Verification items for the finished model (mm, model axes). Face numbers are marked on the shaded views. A direction names the side the tool comes from. Coordinates: 2 decimals unless noted, no trailing zeros. Order: outer loops, then holes, each group sorted by start corner. A loop starts at its lowest first (then second) coordinate and runs counter-clockwise, first axis right, second up. Notation, with made-up numbers: M -8.75,-28 L 34.25,-28 A19 cw 34.25,-8 Z; hole C 2,87 d1. An arc over 180 degrees is marked long. Write item = value, one per line.
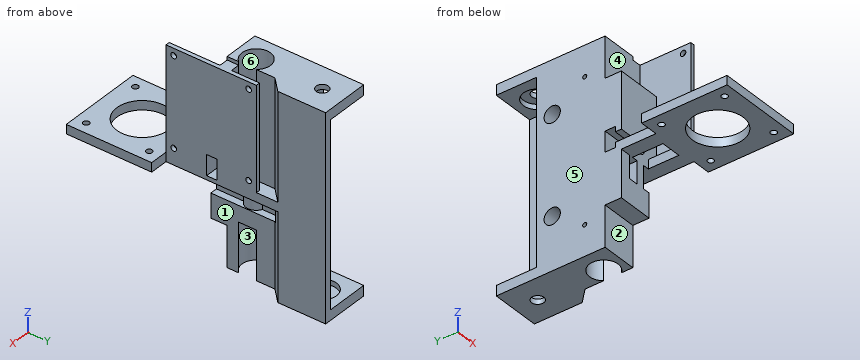
```python
from build123d import *

# Parameters (mm, degrees)
SKETCH1_R               = 7
BOSS_EXTRUDE1_DEPTH     = 50
SKETCH2_R               = 4
CUT_EXTRUDE1_DEPTH      = 17
SKETCH3_W               = 5
SKETCH3_H               = 19.75
BOSS_EXTRUDE2_DEPTH     = 21
SKETCH4_R               = 7
CUT_EXTRUDE4_DEPTH      = 47.5
SKETCH6_R               = 7
SKETCH6_R_2             = 5
BOSS_EXTRUDE3_DEPTH     = 26
CUT_EXTRUDE5_REACH      = 63.576
CUT_EXTRUDE5_END_RADIUS = 7
SKETCH7_R               = 1
CUT_EXTRUDE6_DEPTH      = 102.812634392
CUT_EXTRUDE6_DEPTH_BACK = 102.812634392
SKETCH8_R               = 3
CUT_EXTRUDE7_DEPTH      = 105.209224747
BOSS_EXTRUDE4_DEPTH     = 17.5
CUT_EXTRUDE8_DEPTH      = 78.886134918
SKETCH12_W              = 5
SKETCH12_H              = 11.1
CUT_EXTRUDE9_DEPTH      = 67.234904034
BOSS_EXTRUDE5_REACH     = 82.164
SKETCH13_W              = 6.5
SKETCH13_H              = 4.5
SKETCH14_W              = 2.5
SKETCH14_H              = 5
CUT_EXTRUDE10_DEPTH     = 64.354656605
SKETCH16_R              = 12.5
SKETCH16_R_2            = 1.5
BOSS_EXTRUDE8_DEPTH     = 4.5
SKETCH18_R              = 1.375
BOSS_EXTRUDE9_DEPTH     = 2
BOSS_EXTRUDE10_REACH    = 112.68


with BuildPart() as part:
    # Sketch1 → Boss-Extrude1 (new, symmetric)
    with BuildSketch(Plane.XY):
        Polygon((-12, 7), (9, 7), (9, 26.75), (12, 26.75), (12, -26.75), (-12, -26.75), align=None)
        with Locations((0, -16.75)):
            Circle(SKETCH1_R, mode=Mode.SUBTRACT)
    extrude(amount=BOSS_EXTRUDE1_DEPTH, both=True)

    # Sketch2 → Cut-Extrude1 (cut)
    with BuildSketch(Plane.ZY.offset(12)):
        with Locations((-24.1, -0.75)):
            Circle(SKETCH2_R)
        with Locations((24.1, -0.75)):
            Circle(SKETCH2_R)
    extrude(amount=-CUT_EXTRUDE1_DEPTH, mode=Mode.SUBTRACT)

    # Sketch3 → Boss-Extrude2 (add, through all)
    with BuildSketch(Plane.ZY.offset(-9)):
        with Locations((-47.5, 16.875)):
            Rectangle(SKETCH3_W, SKETCH3_H)
        with Locations((47.5, 16.875)):
            Rectangle(SKETCH3_W, SKETCH3_H)
    extrude(amount=BOSS_EXTRUDE2_DEPTH)

    # Sketch4 → Cut-Extrude4 (cut, symmetric)
    with BuildSketch(Plane.XY):
        with Locations((0, 15.75)):
            Circle(SKETCH4_R)
    extrude(amount=CUT_EXTRUDE4_DEPTH, both=True, mode=Mode.SUBTRACT)

    # Sketch6 → Boss-Extrude3 (add, symmetric)
    with BuildSketch(Plane.XY):
        with Locations((0, -16.75)):
            Circle(SKETCH6_R)
        with Locations(Location((0, -16.75, 0), (0, 0, 180))):
            Circle(SKETCH6_R_2, mode=Mode.SUBTRACT)
    extrude(amount=BOSS_EXTRUDE3_DEPTH, both=True)

    # Cut-Extrude5: up to this cylinder (the profile starts outside it)
    cut_extrude5_end = Plane(origin=(0, -16.75, 0), z_dir=(0, 0, -1)) * Cylinder(CUT_EXTRUDE5_END_RADIUS, 212.152, mode=Mode.PRIVATE)
    # Sketch7 → Cut-Extrude5 (cut, up to the surface)
    with BuildSketch(Plane.ZY.offset(12), mode=Mode.PRIVATE) as cut_extrude5_sk1:
        with Locations((-35, -16.75)):
            Circle(SKETCH7_R)
    cut_extrude5_tool1 = extrude(cut_extrude5_sk1.sketch, amount=-CUT_EXTRUDE5_REACH, mode=Mode.PRIVATE) - cut_extrude5_end
    add(cut_extrude5_tool1.solids().sort_by_distance((-12, -16.75, -35))[0], mode=Mode.SUBTRACT)
    # Sketch7 → Cut-Extrude5 (cut, up to the surface)
    with BuildSketch(Plane.ZY.offset(12), mode=Mode.PRIVATE) as cut_extrude5_sk2:
        with Locations((35, -16.75)):
            Circle(SKETCH7_R)
    cut_extrude5_tool2 = extrude(cut_extrude5_sk2.sketch, amount=-CUT_EXTRUDE5_REACH, mode=Mode.PRIVATE) - cut_extrude5_end
    add(cut_extrude5_tool2.solids().sort_by_distance((-12, -16.75, 35))[0], mode=Mode.SUBTRACT)

    # Sketch8 → Cut-Extrude6 (cut, two sides: drawn at the far end of the back side and taken through both)
    with BuildSketch(Plane(origin=(0, 0, 47.5), x_dir=(-1, 0, 0), z_dir=(0, 0, -1)).offset(-CUT_EXTRUDE6_DEPTH_BACK)):
        with Locations((0, 15.75)):
            Circle(SKETCH8_R)
    extrude(amount=CUT_EXTRUDE6_DEPTH + CUT_EXTRUDE6_DEPTH_BACK, mode=Mode.SUBTRACT)

    # Sketch9 → Cut-Extrude7 (cut, through all)
    with BuildSketch(Plane.XY.offset(50)):
        Polygon((5.5, -3.25), (12, 3.25), (12, -26.75), (5.5, -26.75), align=None)
    extrude(amount=-CUT_EXTRUDE7_DEPTH, mode=Mode.SUBTRACT)

    # Sketch10 → Boss-Extrude4 (add)
    with BuildSketch(Plane.ZY.offset(12)):
        Polygon((-5, -26.75), (-5, -31.75), (5, -31.75), (5, -26.75), (30, -26.75), (30, -34.75), (-30, -34.75), (-30, -26.75), align=None)
    extrude(amount=-BOSS_EXTRUDE4_DEPTH)

    # Sketch11 → Cut-Extrude8 (cut, through all)
    with BuildSketch(Plane(origin=(0, -31.75, 0), x_dir=(1, 0, 0), z_dir=(0, 1, 0))):
        with BuildLine():
            Line((0, 2.5), (-12, 2.5))
            Line((-12, 2.5), (-12, -2.5))
            Line((-12, -2.5), (0, -2.5))
            ThreePointArc((0, -2.5), (2.5, 0), (0, 2.5))
        make_face()
    extrude(amount=-CUT_EXTRUDE8_DEPTH, mode=Mode.SUBTRACT)

    # Sketch12 → Cut-Extrude9 (cut, through all)
    with BuildSketch(Plane(origin=(0, 7, 0), x_dir=(1, 0, 0), z_dir=(0, 1, 0))):
        with Locations((4.5, 12.55)):
            Rectangle(SKETCH12_W, SKETCH12_H)
        with Locations((-4.5, 12.55)):
            Rectangle(SKETCH12_W, SKETCH12_H)
    extrude(amount=-CUT_EXTRUDE9_DEPTH, mode=Mode.SUBTRACT)

    # Sketch13 → Boss-Extrude5 (add, up to next)
    with BuildSketch(Plane.XZ.offset(34.75), mode=Mode.PRIVATE) as boss_extrude5_sk1:
        with Locations((8.75, -4.75)):
            Rectangle(SKETCH13_W, SKETCH13_H)
    boss_extrude5_tool1 = extrude(boss_extrude5_sk1.sketch, amount=-BOSS_EXTRUDE5_REACH, mode=Mode.PRIVATE) - part.part
    add(boss_extrude5_tool1.solids().sort_by_distance((8.75, -34.75, -4.75))[0])

    # Sketch14 → Cut-Extrude10 (cut, through all)
    with BuildSketch(Plane.ZY.offset(-5.5)):
        with Locations((-3.75, -29.25)):
            Rectangle(SKETCH14_W, SKETCH14_H)
    extrude(amount=-CUT_EXTRUDE10_DEPTH, mode=Mode.SUBTRACT)

    # Sketch16 → Boss-Extrude8 (add)
    with BuildSketch(Plane(origin=(0, 0, -7), x_dir=(-1, 0, 0), z_dir=(0, 0, -1))):
        Polygon((-12, -34.75), (-5, -34.75), (-5, -49.75), (5, -49.75), (5, -34.75), (12, -34.75), (12, -51.75), (21, -51.75), (21, -93.75), (-21, -93.75), (-21, -51.75), (-12, -51.75), align=None)
        with Locations((0, -72.75)):
            Circle(SKETCH16_R, mode=Mode.SUBTRACT)
        with Locations((-15.5, -57.25)):
            Circle(SKETCH16_R_2, mode=Mode.SUBTRACT)
        with Locations((15.5, -57.25)):
            Circle(SKETCH16_R_2, mode=Mode.SUBTRACT)
        with Locations((15.5, -88.25)):
            Circle(SKETCH16_R_2, mode=Mode.SUBTRACT)
        with Locations((-15.5, -88.25)):
            Circle(SKETCH16_R_2, mode=Mode.SUBTRACT)
    extrude(amount=-BOSS_EXTRUDE8_DEPTH)

    # Sketch18 → Boss-Extrude9 (add)
    with BuildSketch(Plane(origin=(12, 0, 0), x_dir=(0, 0, -1), z_dir=(1, 0, 0))):
        Polygon((2.5, -51.75), (-48.3, -51.75), (-48.3, -7.3), (2.5, -7.3), (2.5, -26.75), (-5, -26.75), (-5, -31.75), (2.5, -31.75), align=None)
        with Locations((-44.81, -11.11)):
            Circle(SKETCH18_R, mode=Mode.SUBTRACT)
        with Locations((-0.99, -47.94)):
            Circle(SKETCH18_R, mode=Mode.SUBTRACT)
        with Locations((-44.81, -47.94)):
            Circle(SKETCH18_R, mode=Mode.SUBTRACT)
        with Locations((-1.63, -11.11)):
            Circle(SKETCH18_R, mode=Mode.SUBTRACT)
    extrude(amount=-BOSS_EXTRUDE9_DEPTH)

    # Sketch20 → Boss-Extrude10 (add, up to next)
    with BuildSketch(Plane.ZY.offset(-10), mode=Mode.PRIVATE) as boss_extrude10_sk1:
        Polygon((-2.5, -31.75), (-2.5, -34.75), (30, -34.75), (30, -26.75), (48.3, -26.75), (48.3, -21.080127019), (-2.5, -21.080127019), (-2.5, -26.75), (5, -26.75), (5, -31.75), align=None)
    boss_extrude10_tool1 = extrude(boss_extrude10_sk1.sketch, amount=BOSS_EXTRUDE10_REACH, mode=Mode.PRIVATE) - part.part
    add(boss_extrude10_tool1.solids().sort_by_distance((10, -27.004059, 19.830393))[0])


solid = part.part
```
Item 1: Release check for a two-part mould opening along Y. For the marked faces 4, 5 and 6 record: pulls with the +Y half, pulls with the -Y half, needs draft (parallel to the pull), parting line crosses it, or undercut.
Report:
face_4 = pulls with the -Y half
face_5 = needs draft
face_6 = undercut
Item 2: Sectioned sample at C-C, the plane y = -72.75. Enter the section's corners in (x, z).
Report:
outline = M -21,-7 L -12.5,-7 L -12.5,-2.5 L -21,-2.5 Z; M 12.5,-7 L 21,-7 L 21,-2.5 L 12.5,-2.5 Z
Item 3: Sectioned sample at D-D, the plane z = -24.1. Enter the section's corners in (x, y).
Report:
outline = M -12,-34.75 L 5.5,-34.75 L 5.5,-3.25 L 12,3.25 L 12,26.75 L 9,26.75 L 9,7 L -12,7 L -12,3.25 L 5,3.25 L 5,-4.75 L -12,-4.75 Z; hole C 0,-16.75 d10
Item 4: Sectioned sample at B-B, the plane x = -15.5. Enter the section's corners in (y, z), then the cut area to 3 significant figures.
Report:
outline = M -93.75,-7 L -89.75,-7 L -89.75,-2.5 L -93.75,-2.5 Z; M -86.75,-7 L -58.75,-7 L -58.75,-2.5 L -86.75,-2.5 Z; M -55.75,-7 L -51.75,-7 L -51.75,-2.5 L -55.75,-2.5 Z
area = 162 mm^2
Item 5: Tool access check on the marked faces 1, 2 and 3. Record the directions out of +Z, -Z, +X, -X, +Y, -Y that give a thin tool (end or side, any length) a straight path to the whole face; none if there is none.
Report:
face_1 = -Z, +X, -Y
face_2 = -Z, +X, -X, -Y
face_3 = -Z
Item 6: Gauge pin test, flat ends, axial feed: pin 1 (13 mm diameter, centred on y = -0.75, z = -24.1, fed in from +X); pin 2 (12 mm diameter, centred on x = -2, y = -56, fed in from -Z); pin 3 (6 mm diameter, centred on y = -23, z = -36, fed in from -X); pin 4 (8.5 mm diameter, centred on x = 0, y = 15.75, fed in from +Z). Record the tip position at first contact, or that the pin passes through.
Report:
pin_1 = 12
pin_2 = -7
pin_3 = -12
pin_4 = 50
Item 7: Scan lines: L1, parallel to Y at x = 0, z = -3; L2, parallel to Y at x = -15.5, z = -3.8; L3, parallel to Y at x = 11, z = 44. Record each from-to range of solid material in increasing order. Write a range as from..to.
Report:
L1 = -93.75..-85.25, -60.25..-49.75, -34.75..-31.75, -26.75..-21.75, -11.75..7
L2 = -93.75..-89.75, -86.75..-58.75, -55.75..-51.75
L3 = -51.75..-49.05, -46.83..-12.22, -10..-7.3, 2.25..26.75
Item 8: Sectioned sample at A-A, the plane y = 15.75. Enter the section's corners in (x, z).
Report:
outline = M -12,-50 L -3,-50 L -3,-47.5 L -7,-47.5 L -7,-45 L -12,-45 Z; M -12,45 L -7,45 L -7,47.5 L -3,47.5 L -3,50 L -12,50 Z; M 3,-50 L 12,-50 L 12,50 L 3,50 L 3,47.5 L 7,47.5 L 7,45 L 9,45 L 9,-45 L 7,-45 L 7,-47.5 L 3,-47.5 Z
